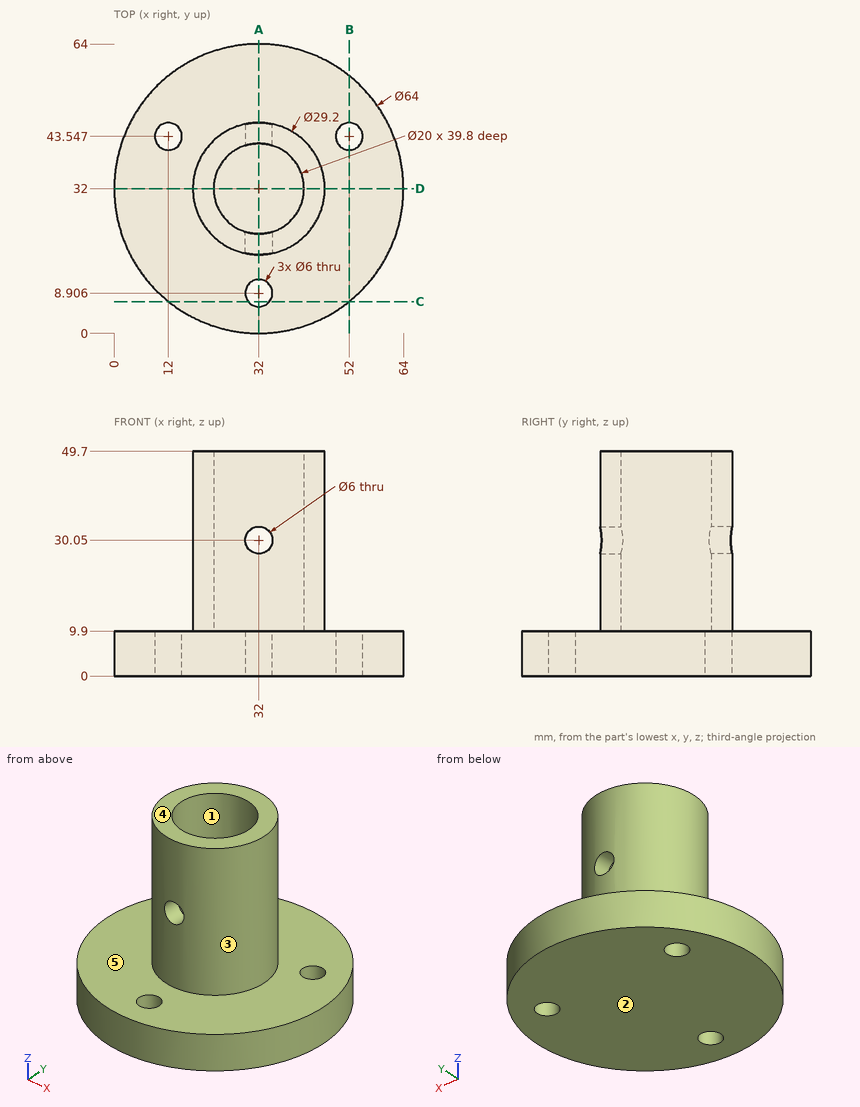
Design review of the part shown in the three views and the two pictorial views. Dimensions are in mm from the part's minimum x, y and z. A direction names the side the tool comes from. Round coordinates to 2 decimals unless told otherwise and drop trailing zeros. Write each loop counter-clockwise with the first axis right and the second up, starting at its lowest first coordinate (ties: lowest second). Pieces come first, ordered by that corner, then holes. Notation, with made-up numbers: (-30.5, 73) -> (7.5, 73) arc R10 ccw to (7.5, 88) -> close; hole circle Ø6 at (30.25, -30). An arc over 180 degrees is marked (long way). Write item = value, one per line. Start each with the question number.
1) Wall thickness on probe 1 along Z at (x, y) = (32, 44.85); probe 2 along Y at (x, z) = (32, 3); probe 3 along Y at (x, z) = (32.5, 44): over which ranges is each line inside the solid? List them lowest first. Write a range as from..to.
2) Take a section at C-C, the plane y = 7. State the section outline as (x, z) points (3 decimals), plus the area to 3 significant figures.
3) Take a section at B-B, the plane x = 52. State the section outline as (y, z) points.
4) Tool access review of the marked faces 4 and 5: name each direction out of +Z, -Z, +X, -X, +Y, -Y from which nothing blocks a thin tool from reaching the whole face with its end or side.
5) Take a section at D-D, the plane y = 32. State the section outline as (x, z) points, plus the area to 4 significant figures.
6) Mouldability with a two-part tool opening along Y and no side actions: class the marked faces 1, 2 and 3 as +Y half, -Y half, draft (parallel to the pull), parting line (faces both ways), or undercut.
7) Clearance check with flat-ended pins moving along their axes: pin 1 (5 mm diameter, centred on x = 32, z = 30.05, fed in from -Y); pin 2 (1 mm diameter, centred on x = 45, z = 8, fed in from -Y); pin 3 (7 mm diameter, centred on x = 32, y = 8.91, fed in from +Z); pin 4 (7 mm diameter, centred on x = 32, z = 30.05, fed in from +Y). State where each tip first meets the part, or that it passes through.
8) Take a section at A-A, the plane x = 32. State the section outline as (y, z) points, plus the area to 3 significant figures.
Results list:
q1.probe_1 = 0..27.05, 33.05..49.7
q1.probe_2 = 0..5.91, 11.91..64
q1.probe_3 = 17.41..22.01, 41.99..46.59
q2.outline = (12.025, 0) -> (29.683, 0) -> (29.683, 9.9) -> (12.025, 9.9) -> close; (34.317, 0) -> (51.975, 0) -> (51.975, 9.9) -> (34.317, 9.9) -> close
q2.area = 350 mm²
q3.outline = (7.02, 0) -> (40.55, 0) -> (40.55, 9.9) -> (7.02, 9.9) -> close; (46.55, 0) -> (56.98, 0) -> (56.98, 9.9) -> (46.55, 9.9) -> close
q4.face_4 = +Z, +X, -X, +Y, -Y
q4.face_5 = +Z
q5.outline = (0, 0) -> (64, 0) -> (64, 9.9) -> (46.6, 9.9) -> (46.6, 49.7) -> (42, 49.7) -> (42, 9.9) -> (22, 9.9) -> (22, 49.7) -> (17.4, 49.7) -> (17.4, 9.9) -> (0, 9.9) -> close
q5.area = 1,000 mm²
q6.face_1 = undercut
q6.face_2 = draft
q6.face_3 = parting line
q7.pin_1 = through
q7.pin_2 = 2.54
q7.pin_3 = 9.9
q7.pin_4 = 46.6
q8.outline = (0, 0) -> (5.91, 0) -> (5.91, 9.9) -> (0, 9.9) -> close; (11.91, 0) -> (64, 0) -> (64, 9.9) -> (46.6, 9.9) -> (46.6, 27.05) -> (42, 27.05) -> (42, 9.9) -> (22, 9.9) -> (22, 27.05) -> (17.4, 27.05) -> (17.4, 9.9) -> (11.91, 9.9) -> close; (17.4, 33.05) -> (22, 33.05) -> (22, 49.7) -> (17.4, 49.7) -> close; (42, 33.05) -> (46.6, 33.05) -> (46.6, 49.7) -> (42, 49.7) -> close
q8.area = 885 mm²
